Drawing for the job (mm, zero at the part's lowest x, y, z). A direction names the side the tool comes from. Coordinates: 2 decimals unless noted, no trailing zeros. Write each loop counter-clockwise with the first axis right and the second up, starting at its lowest first coordinate (ties: lowest second). Pieces come first, ordered by that corner, then holes. Notation, with made-up numbers: M -9,28 L 6,28 A33 cw 6,66 Z; hole C -12.75,-27.5 d6. An arc over 180 degrees is marked long. Use a Markdown table: item, result. Add a question column.
Q1. Slice it at C-C on y = 19. Write the cut outline in (x, z).
Q2. Mould opens along X. For the marked faces 3, 4 and 5 say: released by +X, released by -X, zero draft, split by the parting line, or undercut.
Q3. Tool access for the marked faces 1 and 2: list every direction of +Z, -Z, +X, -X, +Y, -Y with a clear straight run to the whole face (end or side of a thin tool).
Q4. Slice it at B-B on x = 9. Write the cut outline in (y, z).
Q5. Slice it at D-D on x = 17. Write the cut outline in (y, z).
Q6. Slice it at A-A on z = 4.25. Write the cut outline in (x, y), then the cut area to 3 significant figures.
Q7. Pin check, flat tips, straight feed: pin 1 Ø0.9 at (y, z) = (3.5, 1) entering from +X; pin 2 Ø8 at (x, y) = (13.5, 5.5) entering from -Z; pin 3 Ø1.1 at (x, z) = (38.5, 9) entering from -Y; pin 4 Ø2 at (x, z) = (11, 6.5) entering from +Y. Stop position of each tip, or through.
Q8. Wall check: L1, parallel to X at y = 13.5, z = 5.5; L2, parallel to Y at x = 30, z = 1.25; L3, parallel to Y at x = 9, z = 9.1. Give the ranges that are in metal, low to high. Write a range as from..to.
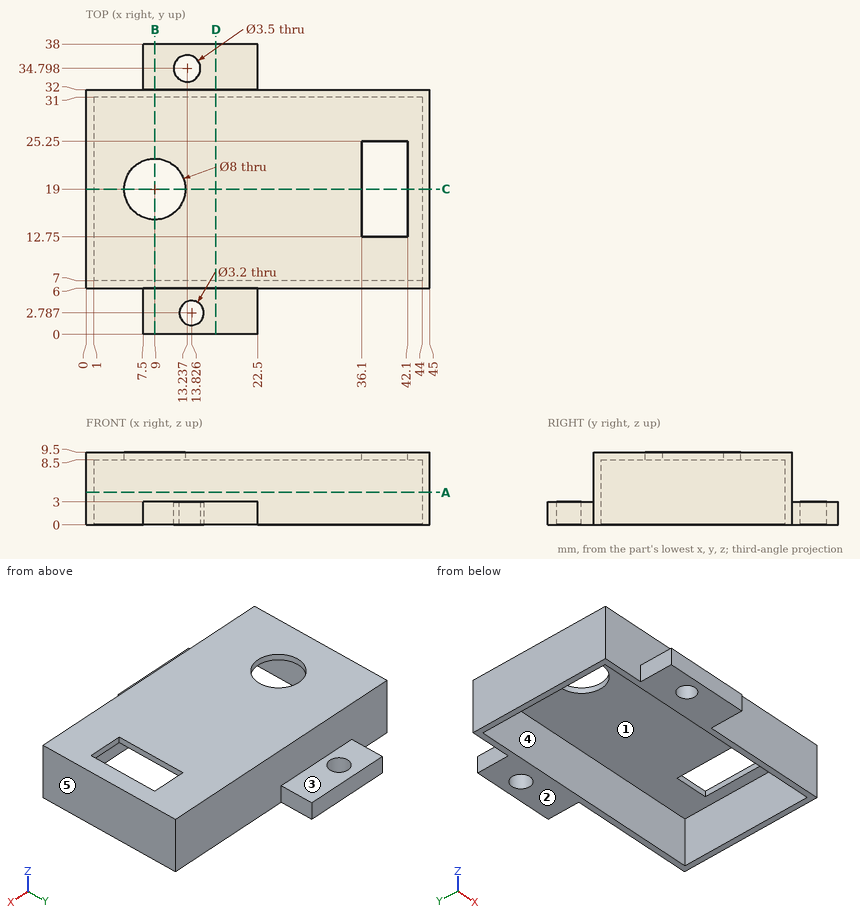
Recorded:
| question | item | result |
|---|---|---|
| 1 | outline | M 0,0 L 1,0 L 1,8.5 L 5,8.5 L 5,9.5 L 0,9.5 Z; M 13,8.5 L 36.1,8.5 L 36.1,9.5 L 13,9.5 Z; M 42.1,8.5 L 44,8.5 L 44,0 L 45,0 L 45,9.5 L 42.1,9.5 Z |
| 2 | face 3 | zero draft |
| 2 | face 4 | undercut |
| 2 | face 5 | released by +X |
| 3 | face 1 | -Z |
| 3 | face 2 | -Z, +X, -X, +Y, -Y |
| 4 | outline | M 0,0 L 7,0 L 7,8.5 L 15,8.5 L 15,9.5 L 6,9.5 L 6,3 L 0,3 Z; M 23,8.5 L 31,8.5 L 31,0 L 38,0 L 38,3 L 32,3 L 32,9.5 L 23,9.5 Z |
| 5 | outline | M 0,0 L 7,0 L 7,8.5 L 31,8.5 L 31,0 L 38,0 L 38,3 L 32,3 L 32,9.5 L 6,9.5 L 6,3 L 0,3 Z |
| 6 | outline | M 0,6 L 45,6 L 45,32 L 0,32 Z; hole M 1,7 L 44,7 L 44,31 L 1,31 Z |
| 6 | area | 138 mm² |
| 7 | pin 1 | x = 22.5 |
| 7 | pin 2 | z = 0 |
| 7 | pin 3 | y = 6 |
| 7 | pin 4 | y = 32 |
| 8 | L1 | 0..1, 44..45 |
| 8 | L2 | 6..7, 31..32 |
| 8 | L3 | 6..15, 23..32 |
